The figure shows three views and two pictorial views of one solid part (mm, origin at its lowest corner). Answer the questions. A direction names the side the tool comes from. Give positions to 0.01 mm unless a question says otherwise; leave off trailing zeros. Order: outer loops, then holes, each group sorted by start corner. A loop starts at its lowest first (then second) coordinate and runs counter-clockwise, first axis right, second up. Notation, with made-up numbers: (22, -11.75) -> (44, -11.75) arc R21 cw to (44, 24.25) -> close; hole circle Ø3 at (-14.75, 29). An arc over 180 degrees is marked (long way). Use one line per item in the form item = value.
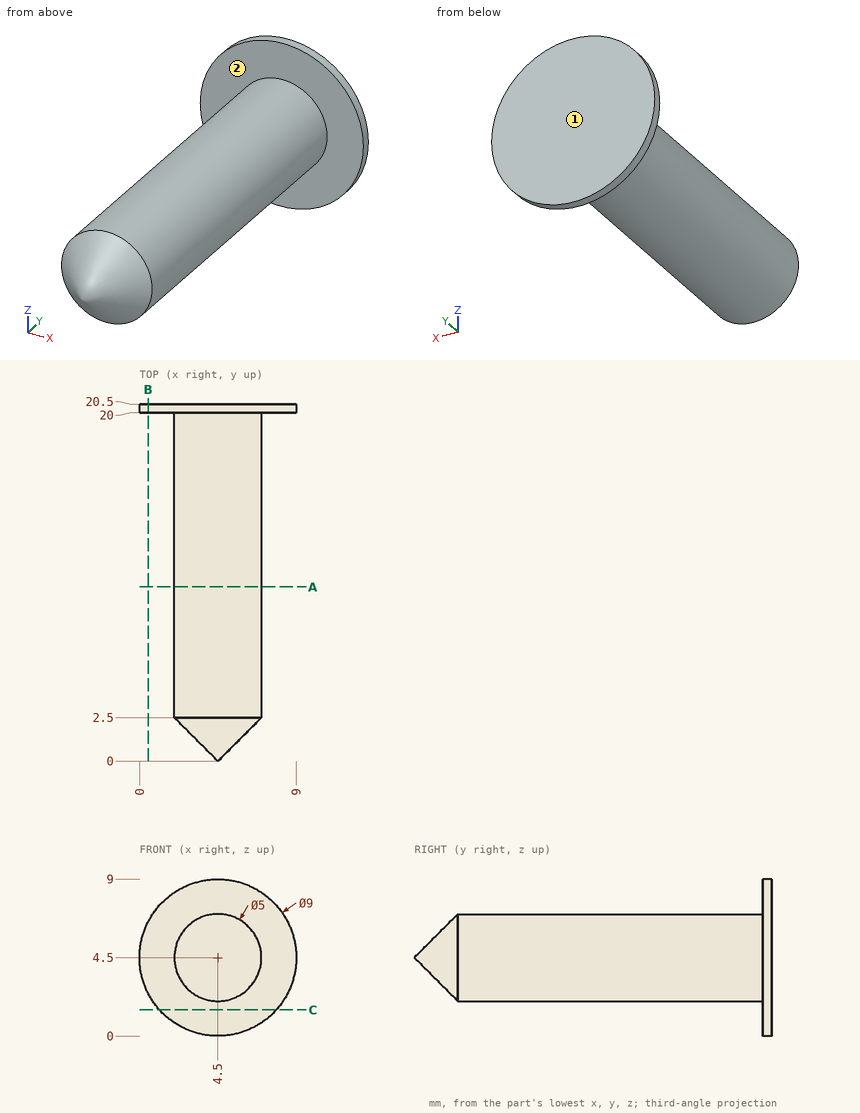
Item 1: The part is cut by section B-B on x = 0.5. Give the vertices of the cut face in (y, z), and give its area (3 significant figures).
Checks:
outline = (20, 2.44) -> (20.5, 2.44) -> (20.5, 6.56) -> (20, 6.56) -> close
area = 2.06 mm²
Item 2: Given pin 1 Ø4.5 at (x, z) = (6.5, 4.5) entering from -Y; pin 2 Ø4 at (y, z) = (4, 7) entering from +X; pin 3 Ø2 at (x, y) = (4, 18) entering from -Z; pin 4 Ø1.5 at (y, z) = (16, 6.5) entering from -X, each flat-ended and moving along its own axis, determine where each tip first touches the part or whether it passes through.
Checks:
pin_1 = 0
pin_2 = 6.95
pin_3 = 2
pin_4 = 2.33
Item 3: The part is cut by section A-A on y = 10. Give the vertices of the cut face in (x, z), and give its area (3 significant figures).
Checks:
outline = circle Ø5 at (4.5, 4.5)
area = 19.6 mm²
Item 4: Which of the six approach directions +Z, -Z, +X, -X, +Y, -Y give full straight-line access (tool end or side, diameter ignored) to the marked faces 1 and 2?
Checks:
face_1 = +Z, -Z, +X, -X, +Y
face_2 = -Y
Item 5: Straight lines are drawn through the part: L1, parallel to Y at x = 3, z = 1.25; L2, parallel to Y at x = 5.75, z = 3.5; L3, parallel to Z at x = 6.75, y = 17.25. For each, find the intervals that lie inside material, in ascending order. Write a range as from..to.
Checks:
L1 = 20..20.5
L2 = 1.6..20.5
L3 = 3.41..5.59
Item 6: The part is cut by section C-C on z = 1.5. Give the vertices of the cut face in (x, y), and give its area (3 significant figures).
Checks:
outline = (1.15, 20) -> (7.85, 20) -> (7.85, 20.5) -> (1.15, 20.5) -> close
area = 3.35 mm²
